from build123d import *

# Parameters (mm, degrees)
BOSS_EXTRUDE1_DEPTH = 3
SKETCH2_R           = 2.05
HEXCUT1_DEPTH       = 3
SKETCH6_R           = 2.05
QUADCUT1_DEPTH      = 3
CUT_EXTRUDE3_DEPTH  = 3
CUT_EXTRUDE4_DEPTH  = 3
SKETCH10_R          = 2.55
HEXBATHOLES_DEPTH   = 3
SKETCH11_R          = 2.55
QUADBATHOLES_DEPTH  = 3
SKETCH13_R          = 1.55
PDBHOLES_DEPTH      = 3
SKETCH15_R          = 1.55
SKETCH15_W          = 40
SKETCH15_H          = 25
CUT_EXTRUDE8_DEPTH  = 3
ACCESSHOLES_DEPTH   = 3


# Read off the part's stored shape, not the designer's step: AccessHoles
with BuildPart() as part:
    # Sketch1 → Boss-Extrude1 (new body)
    with BuildSketch(Plane(origin=(0, 0, 0), x_dir=(1, 0, 0), z_dir=(0, 1, 0))):
        Polygon((150, -40.192378865), (150, 40.192378865), (109.807621135, 109.807621135), (40.192378865, 150), (-40.192378865, 150), (-109.807621135, 109.807621135), (-150, 40.192378865), (-150, -40.192378865), (-109.807621135, -109.807621135), (-40.192378865, -150), (40.192378865, -150), (109.807621135, -109.807621135), align=None)
    extrude(amount=BOSS_EXTRUDE1_DEPTH)

    # Sketch2 → HexCut1 (cut)
    with BuildSketch(Plane(origin=(0, 3, 0), x_dir=(1, 0, 0), z_dir=(0, 1, 0))):
        with Locations(Location((51.014428415, 133.359581934, 0), (0, 0, 270))):
            Circle(SKETCH2_R)
        with Locations(Location((37.344555434, 99.682667397, 0), (0, 0, 270))):
            Circle(SKETCH2_R)
        with Locations(Location((37.344555434, -99.682667397, 0), (0, 0, 270))):
            Circle(SKETCH2_R)
        with Locations(Location((51.014428415, -133.359581934, 0), (0, 0, 270))):
            Circle(SKETCH2_R)
        with Locations(Location((105, 17.5, 0), (0, 0, 270))):
            Circle(SKETCH2_R)
        with Locations(Location((141, 22.5, 0), (0, 0, 270))):
            Circle(SKETCH2_R)
        with Locations(Location((105, -17.5, 0), (0, 0, 270))):
            Circle(SKETCH2_R)
        with Locations(Location((141, -22.5, 0), (0, 0, 270))):
            Circle(SKETCH2_R)
        with Locations(Location((89.985571585, -110.859581934, 0), (0, 0, 270))):
            Circle(SKETCH2_R)
        with Locations(Location((67.655444566, -82.182667397, 0), (0, 0, 270))):
            Circle(SKETCH2_R)
        with Locations(Location((89.985571585, 110.859581934, 0), (0, 0, 270))):
            Circle(SKETCH2_R)
        with Locations(Location((67.655444566, 82.182667397, 0), (0, 0, 270))):
            Circle(SKETCH2_R)
    hexcut1 = extrude(amount=-HEXCUT1_DEPTH, mode=Mode.SUBTRACT)

    # HexCut2: HexCut1 across plane
    add(hexcut1.mirror(Plane(origin=(0, 0, 0), x_dir=(0, 0, 1), z_dir=(1, 0, 0))), mode=Mode.SUBTRACT)

    # Sketch6 → QuadCut1 (cut)
    with BuildSketch(Plane(origin=(0, 3, 0), x_dir=(1, 0, 0), z_dir=(0, 1, 0))):
        with Locations(Location((99.682667397, 37.344555434, 0), (0, 0, 270))):
            Circle(SKETCH6_R)
        with Locations(Location((133.359581934, 51.014428415, 0), (0, 0, 270))):
            Circle(SKETCH6_R)
        with Locations(Location((110.859581934, 89.985571585, 0), (0, 0, 270))):
            Circle(SKETCH6_R)
        with Locations(Location((82.182667397, 67.655444566, 0), (0, 0, 270))):
            Circle(SKETCH6_R)
    quadcut1 = extrude(amount=-QUADCUT1_DEPTH, mode=Mode.SUBTRACT)

    # Mirror1: QuadCut1 across plane
    add(quadcut1.mirror(Plane(origin=(0, 0, 0), x_dir=(0.5000000000000011, 0, 0.8660254037844378), z_dir=(0.8660254037844379, 0, -0.5000000000000012))), mode=Mode.SUBTRACT)

    # Sketch7 → Cut-Extrude3 (cut)
    with BuildSketch(Plane(origin=(0, 3, 0), x_dir=(1, 0, 0), z_dir=(0, 1, 0))):
        with BuildLine():
            Line((46.876606241, 112.192663696), (84.376606241, 177.14456898))
            Line((84.376606241, 177.14456898), (111.223393759, 161.64456898))
            Line((111.223393759, 161.64456898), (73.723393759, 96.692663696))
            ThreePointArc((73.723393759, 96.692663696), (52.55, 91.019269938), (46.876606241, 112.192663696))
        make_face()
        with BuildLine():
            Line((46.876606241, -112.192663696), (84.376606241, -177.14456898))
            Line((84.376606241, -177.14456898), (111.223393759, -161.64456898))
            Line((111.223393759, -161.64456898), (73.723393759, -96.692663696))
            ThreePointArc((73.723393759, -96.692663696), (52.55, -91.019269938), (46.876606241, -112.192663696))
        make_face()
        with BuildLine():
            Line((120.6, 15.5), (160.6, 15.5))
            Line((160.6, 15.5), (160.6, -15.5))
            Line((160.6, -15.5), (120.6, -15.5))
            ThreePointArc((120.6, -15.5), (105.1, 0), (120.6, 15.5))
        make_face()
    cut_extrude3 = extrude(amount=-CUT_EXTRUDE3_DEPTH, mode=Mode.SUBTRACT)

    # Mirror2: Cut-Extrude3 across plane
    add(cut_extrude3.mirror(Plane(origin=(0, 0, 0), x_dir=(0, 0, 1), z_dir=(1, 0, 0))), mode=Mode.SUBTRACT)

    # Sketch8 → Cut-Extrude4 (cut)
    with BuildSketch(Plane(origin=(0, 3, 0), x_dir=(1, 0, 0), z_dir=(0, 1, 0))):
        with BuildLine():
            Line((96.692663696, 73.723393759), (131.333679848, 93.723393759))
            Line((131.333679848, 93.723393759), (146.833679848, 66.876606241))
            Line((146.833679848, 66.876606241), (112.192663696, 46.876606241))
            ThreePointArc((112.192663696, 46.876606241), (91.019269938, 52.55), (96.692663696, 73.723393759))
        make_face()
    cut_extrude4 = extrude(amount=-CUT_EXTRUDE4_DEPTH, mode=Mode.SUBTRACT)

    # Mirror3: Cut-Extrude4 across plane
    add(cut_extrude4.mirror(Plane(origin=(0, 0, 0), x_dir=(0.5000000000000011, 0, 0.8660254037844378), z_dir=(0.8660254037844379, 0, -0.5000000000000012))), mode=Mode.SUBTRACT)

    # Sketch10 → HexBatHoles (cut)
    with BuildSketch(Plane(origin=(0, 3, 0), x_dir=(1, 0, 0), z_dir=(0, 1, 0))):
        with Locations(Location((60, 37.5, 0), (0, 0, 270))):
            Circle(SKETCH10_R)
        with Locations(Location((60, -37.5, 0), (0, 0, 270))):
            Circle(SKETCH10_R)
        with Locations(Location((-60, 37.5, 0), (0, 0, 270))):
            Circle(SKETCH10_R)
        with Locations(Location((-60, -37.5, 0), (0, 0, 270))):
            Circle(SKETCH10_R)
    extrude(amount=-HEXBATHOLES_DEPTH, mode=Mode.SUBTRACT)

    # Sketch11 → QuadBatHoles (cut)
    with BuildSketch(Plane(origin=(0, 3, 0), x_dir=(1, 0, 0), z_dir=(0, 1, 0))):
        with Locations(Location((67.661263769, 20.69307578, 0), (0, 0, 270))):
            Circle(SKETCH11_R)
        with Locations(Location((48.249835386, -51.751361192, 0), (0, 0, 270))):
            Circle(SKETCH11_R)
        with Locations(Location((-67.661263769, -20.69307578, 0), (0, 0, 270))):
            Circle(SKETCH11_R)
        with Locations(Location((-48.249835386, 51.751361192, 0), (0, 0, 270))):
            Circle(SKETCH11_R)
    extrude(amount=-QUADBATHOLES_DEPTH, mode=Mode.SUBTRACT)

    # Sketch13 → PDBHoles (cut)
    with BuildSketch(Plane(origin=(0, 3, 0), x_dir=(1, 0, 0), z_dir=(0, 1, 0))):
        with Locations(Location((-10, 10, 0), (0, 0, 270))):
            Circle(SKETCH13_R)
        with Locations(Location((10, 10, 0), (0, 0, 270))):
            Circle(SKETCH13_R)
        with Locations(Location((-10, -10, 0), (0, 0, 270))):
            Circle(SKETCH13_R)
        with Locations(Location((10, -10, 0), (0, 0, 270))):
            Circle(SKETCH13_R)
    extrude(amount=-PDBHOLES_DEPTH, mode=Mode.SUBTRACT)

    # Sketch15 → Cut-Extrude8 (cut)
    with BuildSketch(Plane(origin=(0, 3, 0), x_dir=(1, 0, 0), z_dir=(0, 1, 0))):
        with Locations((20, -95)):
            Circle(SKETCH15_R)
        with Locations((-20, -95)):
            Circle(SKETCH15_R)
        with Locations((-20, -120)):
            Circle(SKETCH15_R)
        with Locations((20, -120)):
            Circle(SKETCH15_R)
        with Locations((0, -107.5)):
            Rectangle(SKETCH15_W, SKETCH15_H)
        with BuildLine():
            ThreePointArc((-18.45, -95), (-21.096015511, -93.903984489), (-20, -96.55))
            Line((-20, -96.55), (-20, -95))
            Line((-20, -95), (-18.45, -95))
        make_face()
        with BuildLine():
            Line((-20, -95), (-20, -96.55))
            ThreePointArc((-20, -96.55), (-18.903984489, -96.096015511), (-18.45, -95))
            Line((-18.45, -95), (-20, -95))
        make_face()
        with BuildLine():
            ThreePointArc((18.45, -95), (18.903984489, -96.096015511), (20, -96.55))
            Line((20, -96.55), (20, -95))
            Line((20, -95), (18.45, -95))
        make_face()
        with BuildLine():
            Line((20, -95), (20, -96.55))
            ThreePointArc((20, -96.55), (21.096015511, -96.096015511), (21.55, -95))
            ThreePointArc((21.55, -95), (20, -93.45), (18.45, -95))
            Line((18.45, -95), (20, -95))
        make_face()
        with BuildLine():
            ThreePointArc((20, -118.45), (18.903984489, -118.903984489), (18.45, -120))
            Line((18.45, -120), (20, -120))
            Line((20, -120), (20, -118.45))
        make_face()
        with BuildLine():
            Line((20, -120), (18.45, -120))
            ThreePointArc((18.45, -120), (20, -121.55), (21.55, -120))
            ThreePointArc((21.55, -120), (21.096015511, -118.903984489), (20, -118.45))
            Line((20, -118.45), (20, -120))
        make_face()
        with BuildLine():
            Line((-20, -118.45), (-20, -120))
            Line((-20, -120), (-18.45, -120))
            ThreePointArc((-18.45, -120), (-18.903984489, -118.903984489), (-20, -118.45))
        make_face()
        with BuildLine():
            Line((-18.45, -120), (-20, -120))
            Line((-20, -120), (-20, -118.45))
            ThreePointArc((-20, -118.45), (-21.096015511, -121.096015511), (-18.45, -120))
        make_face()
    extrude(amount=-CUT_EXTRUDE8_DEPTH, mode=Mode.SUBTRACT)

    # AccessHoles outline → AccessHoles (cut)
    with BuildSketch(Plane(origin=(0, 0, 0), x_dir=(1, 0, 0), z_dir=(0, 1, 0))):
        with BuildLine():
            ThreePointArc((-18.45, 123.640367336), (-21.096015511, 124.736382847), (-20, 122.090367336))
            Line((-20, 122.090367336), (-20, 100.190367336))
            ThreePointArc((-20, 100.190367336), (-21.096015511, 97.544351825), (-18.45, 98.640367336))
            Line((-18.45, 98.640367336), (18.45, 98.640367336))
            ThreePointArc((18.45, 98.640367336), (21.096015511, 97.544351825), (20, 100.190367336))
            Line((20, 100.190367336), (20, 122.090367336))
            ThreePointArc((20, 122.090367336), (21.096015511, 124.736382847), (18.45, 123.640367336))
            Line((18.45, 123.640367336), (-18.45, 123.640367336))
        make_face()
        with BuildLine():
            ThreePointArc((114.72437375, -43.111739466), (116.996558781, -41.36823057), (114.157034374, -40.99440009))
            Line((114.157034374, -40.99440009), (95.191078031, -30.04440009))
            ThreePointArc((95.191078031, -30.04440009), (93.447569135, -27.77221506), (93.073738655, -30.611739466))
            Line((93.073738655, -30.611739466), (74.623738655, -62.568076866))
            ThreePointArc((74.623738655, -62.568076866), (72.351553625, -64.311585762), (75.191078031, -64.685416242))
            Line((75.191078031, -64.685416242), (94.157034374, -75.635416242))
            ThreePointArc((94.157034374, -75.635416242), (95.90054327, -77.907601273), (96.27437375, -75.068076866))
            Line((96.27437375, -75.068076866), (114.72437375, -43.111739466))
        make_face()
        with BuildLine():
            ThreePointArc((-74.623738655, 66.208444202), (-72.351553625, 67.951953098), (-75.191078031, 68.325783577))
            Line((-75.191078031, 68.325783577), (-94.157034374, 79.275783577))
            ThreePointArc((-94.157034374, 79.275783577), (-95.900543269, 81.547968608), (-96.27437375, 78.708444202))
            Line((-96.27437375, 78.708444202), (-114.72437375, 46.752106802))
            ThreePointArc((-114.72437375, 46.752106802), (-116.996558781, 45.008597906), (-114.157034374, 44.634767426))
            Line((-114.157034374, 44.634767426), (-95.191078031, 33.684767426))
            ThreePointArc((-95.191078031, 33.684767426), (-93.447569135, 31.412582395), (-93.073738655, 34.252106802))
            Line((-93.073738655, 34.252106802), (-74.623738655, 66.208444202))
        make_face()
    extrude(amount=ACCESSHOLES_DEPTH, mode=Mode.SUBTRACT)


solid = part.part
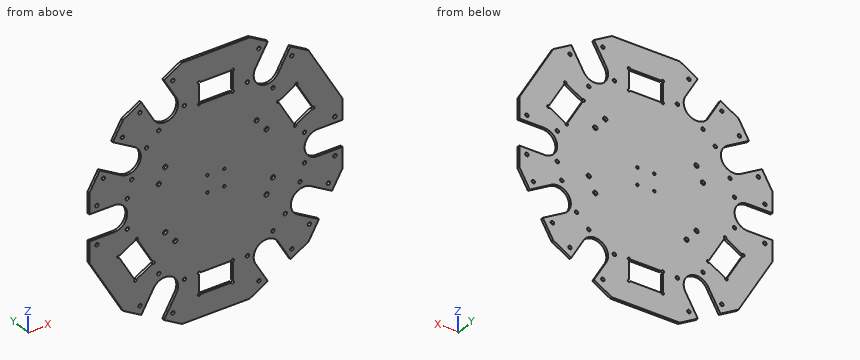
Could you check a few things on this model? Use its own coordinates, in mm. Give positions to 0.01 mm unless a question says otherwise; leave off trailing zeros. Answer in a Markdown table with one row per item. Add a question column.
Item 1: Imagine slicing it at A-A (y = 0.6). Count the separate pieces of the cut face and the enclosed holes in it, and give its area (3 significant figures).
Item 2: Please list where these lines run through material, in increasing order: probe 1 along Z at (x, y) = (-6.5, 2.7); probe 2 along Z at (x, y) = (55, 1.5); probe 3 along X at (y, z) = (2.5, 17).
Item 3: I'm going to push flat-ended pins straight in: P1, Ø10, axis at x = 53.5, z = 105, coming from the -Y side; P2, Ø1, axis at x = -49, y = 2, coming from the -Z side; P3, Ø1, axis at x = 113.5, y = 2, coming from the -Z side. Where does each tip first touch, or does it pass through?
Result:
| question | item | result |
|---|---|---|
| 1 | separate pieces | 1 |
| 1 | enclosed holes | 48 |
| 1 | area | 57,300 mm2 |
| 2 | probe 1 | -150 to -123.64, -98.64 to 95, 120 to 150 |
| 2 | probe 2 | -141.45 to -126.26, -89.88 to 89.88, 126.26 to 141.45 |
| 2 | probe 3 | -150 to -106.99, -103.01 to 103.01, 106.99 to 150 |
| 3 | P1 | through |
| 3 | P2 | z = -145.2 |
| 3 | P3 | z = -104.28 |
